Autodesk Inventor part; units mm, degrees
ref_plane "Work Plane1" through (6.985, 0, 0) normal (1, 0, 0) x (0, 1, 0)
ref_plane "Work Plane2" through (0, 0, 0) normal (0.7071, 0, -0.7071) x (0, 1, 0)
ref_plane "XZ Plane" through (0, 0, 0) normal (0, 1, 0) x (-1, 0, 0)
sketch "Sketch1" plane through (0, 0, 0) normal (0, 1, 0) x (-1, 0, 0)
  circle A0 centre (0, 0) radius 4.8895
  circle A1 centre (0, 0) radius 6.985
  dimension "d0" = 9.779
  dimension "d1" = 13.97
extrude "Extrusion1" add sketch "Sketch1" along normal blind 6.35
ref_plane "Work Plane1" through (6.985, 0, 0) normal (1, 0, 0) x (0, 1, 0)
sketch "Sketch2" plane through (6.985, 0, 0) normal (1, 0, 0) x (0, 1, 0)
  circle A0 centre (3.175, 0) radius 1.905
  line L0 (0, -6.985) -> (6.35, -6.985)
  point P0 (0, 0)
  point P1 (3.175, -6.985)
  dimension "d4" = 3.81
extrude "Extrusion2" cut sketch "Sketch2" against normal blind 6.35
ref_plane "Work Plane2" through (0, 0, 0) normal (0.7071, 0, -0.7071) x (0, 1, 0)
sketch "Sketch4" plane through (0, 0, 0) normal (0.7071, 0, -0.7071) x (0, 1, 0)
  circle A0 centre (3.175, 0) radius 1.7145
  line L0 (0, -6.985) -> (6.35, -6.985)
  point P0 (0, 0)
  point P1 (3.175, -6.985)
  dimension "d11" = 3.429
extrude "Extrusion4" cut sketch "Sketch4" along normal through all both and the other way through all
pattern_circular "Circular Pattern1" count 2 over 90 about axis through (0, 0, 0) along (0, 1, 0) of "Extrusion4"
properties part number "SpoolCarrageMagnetMount" material "ABS Plastic"
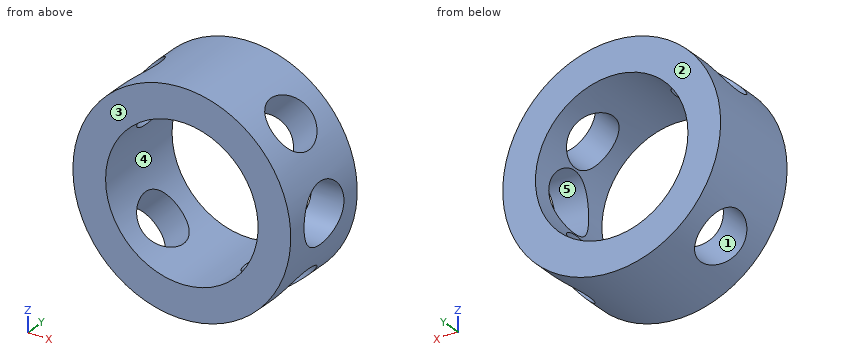
Verification items for the finished model (mm, model axes). Face numbers are marked on the shaded views. A direction names the side the tool comes from. Round coordinates to 2 decimals unless told otherwise and drop trailing zeros. Order: outer loops, then holes, each group sorted by start corner. A loop starts at its lowest first (then second) coordinate and runs counter-clockwise, first axis right, second up.
1) Material ranges on line 1 (Z direction, x = 0, y = 1.75) (1 decimal); line 2 (Y direction, x = -4.5, z = 3.25); line 3 (X direction, y = 0.5, z = 4.5), recorded low to high.
Geometry says:
line 1: z = -7 to -4.9, 4.9 to 7
line 2: y = 0 to 1.71, 4.64 to 6.35
line 3: x = -5.34 to -1.91, 1.91 to 5.34
2) Cross-section at A-A, the plane z = 0. Give the number of separate pieces and of enclosed holes in the cut face, plus the area to 3 significant figures.
Geometry says:
separate pieces: 3
enclosed holes: 0
area: 18.6 mm2
3) Draft check along Y on the marked faces 1, 2 and 3. Enter one of: +Y half, -Y half, draft (parallel to the pull), parting line (faces both ways), or undercut.
Geometry says:
face 1: undercut
face 2: +Y half
face 3: -Y half
4) Tool access check on the marked faces 4 and 5. Record the directions out of +Z, -Z, +X, -X, +Y, -Y that give a thin tool (end or side, any length) a straight path to the whole face; none if there is none.
Geometry says:
face 4: +Y, -Y
face 5: +X
5) Cross-section at D-D, the plane y = 1. Record the cut outline in (x, z) (1 decimal).
Geometry says:
outline: circle Ø14 at (0, 0); hole circle Ø9.8 at (0, 0)
6) Depth check by flat-ended pin: pin 1 (1.5 mm diameter, centred on y = 5.5, z = -1, fed in from -X); pin 2 (1 mm diameter, centred on x = -4.5, y = 1, fed in from +Z). Enter the tip coordinate at first touch or a pass-through.
Geometry says:
pin 1: stops at x = -6.98
pin 2: stops at z = 5.73
